from build123d import *

# Parameters (mm, degrees)
SKETCH4_W                                  = 42
SKETCH4_H                                  = 42
SKETCH4_R                                  = 1.6
BOSS_EXTRUDE1_DEPTH                        = 1.5
SKETCH5_R                                  = 12
CUT_EXTRUDE1_DEPTH                         = 30.736341402
BOSS_EXTRUDE2_DEPTH                        = 2
SKETCH7_W                                  = 46
SKETCH7_H                                  = 43.5
BOSS_EXTRUDE3_DEPTH                        = 2
CUT_EXTRUDE2_DEPTH                         = 0.2
SKETCH9_W                                  = 42.4
SKETCH9_H                                  = 42
CUT_EXTRUDE3_DEPTH                         = 0.2
BOSS_EXTRUDE4_DEPTH                        = 43.5
SKETCH16_W                                 = 10
SKETCH16_H                                 = 5
CUT_EXTRUDE6_DEPTH                         = 12
SKETCH12_R                                 = 1.6
CUT_EXTRUDE8_DEPTH                         = 65.209004806
SKETCH18_R                                 = 3.6
CUT_EXTRUDE9_DEPTH                         = 1.5
MIRROR7_AT_THE_SECOND_PLANE_COPY_1_SKETC_R = 3.6
MIRROR7_AT_THE_SECOND_PLANE_COPY_1_DEPTH   = 1.5
CUT_EXTRUDE10_REACH                        = 66.209
CUT_EXTRUDE10_END_RADIUS                   = 85
SKETCH22_R                                 = 1.6


with BuildPart() as part:
    # Sketch4 → Boss-Extrude1 (new body)
    with BuildSketch(Plane(origin=(0, 0, 0), x_dir=(1, 0, 0), z_dir=(0, 1, 0))):
        Rectangle(SKETCH4_W, SKETCH4_H)
        with Locations(Location((-15.4, 15.4, 0), (0, 0, 270))):
            Circle(SKETCH4_R, mode=Mode.SUBTRACT)
        with Locations(Location((15.4, 15.4, 0), (0, 0, 90))):
            Circle(SKETCH4_R, mode=Mode.SUBTRACT)
        with Locations(Location((15.4, -15.4, 0), (0, 0, 270))):
            Circle(SKETCH4_R, mode=Mode.SUBTRACT)
        with Locations(Location((-15.4, -15.4, 0), (0, 0, 90))):
            Circle(SKETCH4_R, mode=Mode.SUBTRACT)
    extrude(amount=BOSS_EXTRUDE1_DEPTH)

    # Sketch5 → Cut-Extrude1 (cut, through all)
    with BuildSketch(Plane(origin=(0, 1.5, 0), x_dir=(1, 0, 0), z_dir=(0, 1, 0))):
        with Locations(Location((0, 0, 0), (0, 0, 270))):
            Circle(SKETCH5_R)
    extrude(amount=-CUT_EXTRUDE1_DEPTH, mode=Mode.SUBTRACT)

    # Sketch6 → Boss-Extrude2 (add)
    with BuildSketch(Plane(origin=(21, 0, 0), x_dir=(0, 0, -1), z_dir=(1, 0, 0))):
        Polygon((-21, 0), (21, -42), (21, 0), (21, 1.5), (-21, 1.5), align=None)
    boss_extrude2 = extrude(amount=BOSS_EXTRUDE2_DEPTH)

    # Mirror1: Boss-Extrude2 across plane
    add(boss_extrude2.mirror(Plane(origin=(0, 0, 0), x_dir=(0, 0, 1), z_dir=(1, 0, 0))))

    # Sketch7 → Boss-Extrude3 (add)
    with BuildSketch(Plane(origin=(0, 0, -21), x_dir=(-1, 0, 0), z_dir=(0, 0, -1))):
        with Locations((0, -20.25)):
            Rectangle(SKETCH7_W, SKETCH7_H)
    extrude(amount=BOSS_EXTRUDE3_DEPTH)

    # Sketch8 → Cut-Extrude2 (cut)
    with BuildSketch(Plane(origin=(-21, 0, 0), x_dir=(0, 0, -1), z_dir=(1, 0, 0))):
        Polygon((-21, 0), (21, -42), (21, 0), align=None)
    cut_extrude2 = extrude(amount=-CUT_EXTRUDE2_DEPTH, mode=Mode.SUBTRACT)

    # Mirror2: Cut-Extrude2 across plane
    add(cut_extrude2.mirror(Plane(origin=(0, 0, 0), x_dir=(0, 0, 1), z_dir=(1, 0, 0))), mode=Mode.SUBTRACT)

    # Sketch9 → Cut-Extrude3 (cut)
    with BuildSketch(Plane.XY.offset(-21)):
        with Locations((0, -21)):
            Rectangle(SKETCH9_W, SKETCH9_H)
    extrude(amount=-CUT_EXTRUDE3_DEPTH, mode=Mode.SUBTRACT)

    # Sketch14 → Boss-Extrude4 (add)
    with BuildSketch(Plane(origin=(0, 1.5, 0), x_dir=(1, 0, 0), z_dir=(0, 1, 0))):
        with BuildLine():
            Line((-23, 23), (23, 23))
            Line((23, 23), (24.040721666, 26.529403909))
            ThreePointArc((24.040721666, 26.529403909), (0, 30), (-24.040721666, 26.529403909))
            Line((-24.040721666, 26.529403909), (-23, 23))
        make_face()
    extrude(amount=-BOSS_EXTRUDE4_DEPTH)

    # Sketch16 → Cut-Extrude6 (cut)
    with BuildSketch(Plane.XZ.offset(42)):
        with Locations((0, -23.7)):
            Rectangle(SKETCH16_W, SKETCH16_H)
    extrude(amount=-CUT_EXTRUDE6_DEPTH, mode=Mode.SUBTRACT)

    # Sketch12 → Cut-Extrude8 (cut, through all)
    with BuildSketch(Plane.XY.offset(-21.2)):
        with Locations((16.4, -4.6)):
            Circle(SKETCH12_R)
    extrude(amount=-CUT_EXTRUDE8_DEPTH, mode=Mode.SUBTRACT)

    # Sketch18 → Cut-Extrude9 (cut)
    with BuildSketch(Plane.XY.offset(-21.2)):
        with Locations((16.4, -4.6)):
            Circle(SKETCH18_R)
    cut_extrude9 = extrude(amount=-CUT_EXTRUDE9_DEPTH, mode=Mode.SUBTRACT)

    # Mirror7: Cut-Extrude9 across plane
    add(cut_extrude9.mirror(Plane(origin=(0, -21, 0), x_dir=(0, 0, 1), z_dir=(0, -1, 0))), mode=Mode.SUBTRACT)

    # Mirror7 at the second plane: Cut-Extrude9 across plane
    add(cut_extrude9.mirror(Plane(origin=(0, 0, 0), x_dir=(0, 0, 1), z_dir=(1, 0, 0))), mode=Mode.SUBTRACT)

    # Mirror7 at the second plane copy 1 sketc → Mirror7 at the second plane copy 1 (cut)
    with BuildSketch(Plane(origin=(0, -42, -21.2), x_dir=(-1, 0, 0), z_dir=(0, 0, 1))):
        with Locations((16.4, -4.6)):
            Circle(MIRROR7_AT_THE_SECOND_PLANE_COPY_1_SKETC_R)
    extrude(amount=-MIRROR7_AT_THE_SECOND_PLANE_COPY_1_DEPTH, mode=Mode.SUBTRACT)

    # Cut-Extrude10: up to this cylinder (the profile starts inside it)
    cut_extrude10_end = Plane(origin=(0, -21, 55), z_dir=(0, 1, 0)) * Cylinder(CUT_EXTRUDE10_END_RADIUS, 336.218, mode=Mode.PRIVATE)
    # Sketch22 → Cut-Extrude10 (cut, up to the surface)
    with BuildSketch(Plane.XY.offset(-21.2), mode=Mode.PRIVATE) as cut_extrude10_sk1:
        with Locations((-16.4, -37.4)):
            Circle(SKETCH22_R)
    cut_extrude10_tool1 = extrude(cut_extrude10_sk1.sketch, amount=-CUT_EXTRUDE10_REACH, mode=Mode.PRIVATE) & cut_extrude10_end
    add(cut_extrude10_tool1.solids().sort_by_distance((-16.4, -37.4, -21.2))[0], mode=Mode.SUBTRACT)
    # Sketch22 → Cut-Extrude10 (cut, up to the surface)
    with BuildSketch(Plane.XY.offset(-21.2), mode=Mode.PRIVATE) as cut_extrude10_sk2:
        with Locations((-16.4, -4.6)):
            Circle(SKETCH22_R)
    cut_extrude10_tool2 = extrude(cut_extrude10_sk2.sketch, amount=-CUT_EXTRUDE10_REACH, mode=Mode.PRIVATE) & cut_extrude10_end
    add(cut_extrude10_tool2.solids().sort_by_distance((-16.4, -4.6, -21.2))[0], mode=Mode.SUBTRACT)
    # Sketch22 → Cut-Extrude10 (cut, up to the surface)
    with BuildSketch(Plane.XY.offset(-21.2), mode=Mode.PRIVATE) as cut_extrude10_sk3:
        with Locations((16.4, -37.4)):
            Circle(SKETCH22_R)
    cut_extrude10_tool3 = extrude(cut_extrude10_sk3.sketch, amount=-CUT_EXTRUDE10_REACH, mode=Mode.PRIVATE) & cut_extrude10_end
    add(cut_extrude10_tool3.solids().sort_by_distance((16.4, -37.4, -21.2))[0], mode=Mode.SUBTRACT)


solid = part.part
For this review, take the finished solid that the model builds, in its own axes (mm). A direction names the side the tool comes from. Round coordinates to 2 decimals unless told otherwise and drop trailing zeros. Loops run counter-clockwise (first coordinate to the right, second up) from the corner with the lowest first, then second, coordinate; pieces in that order, holes last. Notation, with made-up numbers: (6.25, -34.5) - (13.25, -34.5) arc R8 cw to (13.25, -22.5) - close; hole circle Ø2 at (68.25, 72). An arc over 180 degrees is marked (long way). Answer as CSV lines item,"result".
(1) Mouldability with a two-part tool opening along X and no side actions: class faces 1 (the face through (-14.79, 0.74, 13.92)), 2 (the face through (23, -16, -6)), 3 (the face through (0, -20, -30)), 4 (the face through (14.79, 0.74, 16.88)) as +X half, -X half, draft (parallel to the pull), parting line (faces both ways), or undercut.
Checked values:
face 1,"undercut"
face 2,"+X half"
face 3,"parting line"
face 4,"undercut"
(2) Consider section B-B on x = 0. Give the boundary of the cut face in (y, z), then the cut area to 3 significant figures.
Checked values:
outline,"(-42, -30) - (1.5, -30) - (1.5, -12) - (0, -12) - (0, -21.2) - (-30, -21.2) - (-30, -26.2) - (-42, -26.2) - close; (0, 12) - (1.5, 12) - (1.5, 21) - (0, 21) - close"
area,"350 mm2"
(3) Consider section A-A on z = 15.4. Give the boundary of the cut face in (x, y), then the cut area to 3 significant figures.
Checked values:
outline,"(-23, -5.6) - (-21.2, -5.6) - (-21.2, 0) - (-17, 0) - (-17, 1.5) - (-23, 1.5) - close; (-13.8, 0) - (13.8, 0) - (13.8, 1.5) - (-13.8, 1.5) - close; (17, 0) - (21.2, 0) - (21.2, -5.6) - (23, -5.6) - (23, 1.5) - (17, 1.5) - close"
area,"79.6 mm2"
(4) Consider section C-C on z = 0. Give the boundary of the cut face in (x, y).
Checked values:
outline,"(-23, -21) - (-21.2, -21) - (-21.2, 0) - (-12, 0) - (-12, 1.5) - (-23, 1.5) - close; (12, 0) - (21.2, 0) - (21.2, -21) - (23, -21) - (23, 1.5) - (12, 1.5) - close"
(5) Consider section D-D on y = -4.6. Give the boundary of the cut face in (x, z).
Checked values:
outline,"(-24.04, -26.53) arc R85 ccw to (-18, -28.07) - (-18, -22.7) - (-20, -22.7) - (-20, -21.2) - (-21.2, -21.2) - (-21.2, 16.4) - (-23, 16.4) - (-23, -23) - close; (-14.8, -28.7) arc R85 ccw to (14.8, -28.7) - (14.8, -22.7) - (12.8, -22.7) - (12.8, -21.2) - (-12.8, -21.2) - (-12.8, -22.7) - (-14.8, -22.7) - close; (18, -28.07) arc R85 ccw to (24.04, -26.53) - (23, -23) - (23, 16.4) - (21.2, 16.4) - (21.2, -21.2) - (20, -21.2) - (20, -22.7) - (18, -22.7) - close"
(6) Tool access review of faces 5 (the face through (5, -36, -24)), 6 (the face through (-17.95, -3.75, -22.7)), 7 (the face through (0, 1.5, -16)): name each direction out of +Z, -Z, +X, -X, +Y, -Y from which nothing blocks a thin tool from reaching the whole face with its end or side.
Checked values:
face 5,"+Z, -Y"
face 6,"+Z"
face 7,"+Z, -Z, +X, -X, +Y"
(7) Insertion check: P1, Ø6, axis at x = -8.5, y = -22.5, coming from the +Z side; P2, Ø1.5, axis at x = -3, y = -13.5, coming from the -Z side; P3, Ø2, axis at x = 17.5, y = -37, coming from the +Z side; P4, Ø2.5, axis at x = 16.4, y = -4.6, coming from the +Z side. Each pin has a flat end and moves straight along its axis. Give the tip position at first contact, or say it passes through.
Checked values:
P1,"stops at z = -21.2"
P2,"stops at z = -29.97"
P3,"stops at z = -22.7"
P4,"passes through"
(8) Wall thickness on line 1 (X direction, y = 0.9, z = -15.4); line 2 (Y direction, x = 16.4, z = -24.25); line 3 (Y direction, x = -16.4, z = -21.75): over which ranges is each line inside the solid? List them lowest first.
Checked values:
line 1,"x = -23 to -17, -13.8 to 13.8, 17 to 23"
line 2,"y = -42 to -39, -35.8 to -6.2, -3 to 1.5"
line 3,"y = -42 to -41, -33.8 to -8.2, -1 to 1.5"
